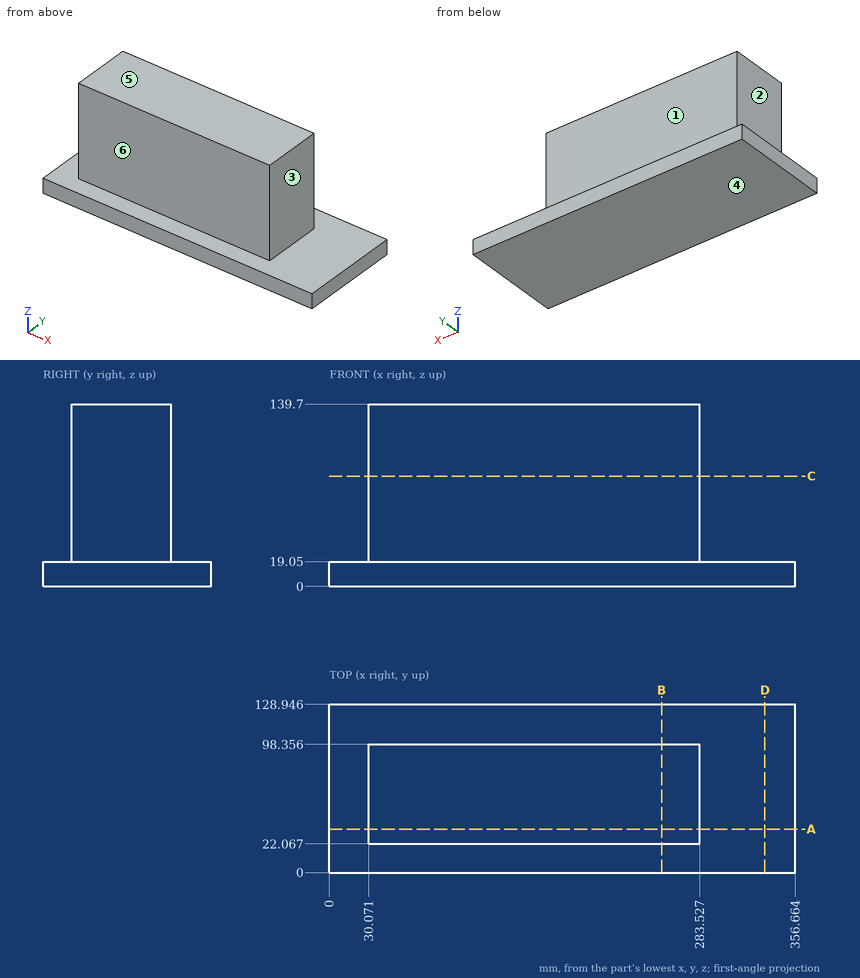
The figure shows three views and two pictorial views of one solid part (mm, origin at its lowest corner). Answer the questions. A direction names the side the tool comes from. Round coordinates to 2 decimals unless told otherwise and drop trailing zeros. Write each loop counter-clockwise with the first axis right and the second up, starting at its lowest first coordinate (ties: lowest second). Pieces come first, ordered by that corner, then holes. Notation, with made-up numbers: (18, -39) -> (26, -39) arc R29 cw to (26, -14) -> close; hole circle Ø4 at (68.5, -15.5). An arc over 180 degrees is marked (long way). Answer as a JSON object with one key per item and string values. Group by question number.
Q1. Which of the six approach directions +Z, -Z, +X, -X, +Y, -Y give full straight-line access (tool end or side, diameter ignored) to the marked faces 1, 2 and 3?
Q2. Section B-B (x = 254.5) is taken. Write down the section's boundary in (y, z), plus the area to 3 significant figures.
Q3. Each of these flat-tipped pins is pushed along its axis until it touches: pin 1 Ø1.5 at (y, z) = (22, 74.5) entering from +X; pin 2 Ø10 at (x, z) = (93.5, 80.5) entering from -Y; pin 3 Ø2 at (x, z) = (166, 43.5) entering from +Y. Where does it stop, or does it pass through?
Q4. Straight lines are drawn through the part: line 1 along Y through (x, z) = (38.5, 128.5); line 2 along X through (y, z) = (67.5, 113.5); line 3 along Z through (x, y) = (231.5, 115). For each, find the intervals that lie inside material, in ascending order.
Q5. Determine the mould class of the marked faces 4, 5 and 6 for opening direction Z: pulls with the +Z half, pulls with the -Z half, needs draft (parallel to the pull), parting line crosses it, or undercut.
Q6. Section A-A (y = 33.5) is taken. Write down the section's boundary in (x, z), plus the area to 3 significant figures.
Q7. Section C-C (z = 84.5) is taken. Write down the section's boundary in (x, y).
Q8. Section D-D (x = 333.5) is taken. Write down the section's boundary in (y, z).
Check values:
{
 "1": {"face 1": "+Z, +X, -X, +Y", "face 2": "+Z, -X, +Y, -Y", "face 3": "+Z, +X, +Y, -Y"},
 "2": {"outline": "(0, 0) -> (128.95, 0) -> (128.95, 19.05) -> (98.36, 19.05) -> (98.36, 139.7) -> (22.07, 139.7) -> (22.07, 19.05) -> (0, 19.05) -> close", "area": "11,700 mm^2"},
 "3": {"pin 1": "x = 283.53", "pin 2": "y = 22.07", "pin 3": "y = 98.36"},
 "4": {"line 1": "22.07 to 98.36", "line 2": "30.07 to 283.53", "line 3": "0 to 19.05"},
 "5": {"face 4": "pulls with the -Z half", "face 5": "pulls with the +Z half", "face 6": "needs draft"},
 "6": {"outline": "(0, 0) -> (356.66, 0) -> (356.66, 19.05) -> (283.53, 19.05) -> (283.53, 139.7) -> (30.07, 139.7) -> (30.07, 19.05) -> (0, 19.05) -> close", "area": "37,400 mm^2"},
 "7": {"outline": "(30.07, 22.07) -> (283.53, 22.07) -> (283.53, 98.36) -> (30.07, 98.36) -> close"},
 "8": {"outline": "(0, 0) -> (128.95, 0) -> (128.95, 19.05) -> (0, 19.05) -> close"}
}
